```python
from build123d import *

# Parameters (mm, degrees)
EXTRUDE_1_DEPTH     = 5
FILLET_1_R          = 2.5
FILLET_2_R          = 1
EXTRUDE_2_DEPTH     = 8
FILLET_3_R          = 2.5
SKETCH_5_W          = 1.467751534
SKETCH_5_H          = 4.178210798
SKETCH_5_W_2        = 1.389566385
CUT_EXTRUDE_1_DEPTH = 20
FILLET_4_R          = 1.5
FILLET_5_R          = 1.5


with BuildPart() as part:
    # 草图1 → 凸台-拉伸1 (new body)
    with BuildSketch(Plane.XY):
        Polygon((0, 0), (0, 28), (4, 28), (7.380946094, 20.749537704), (11.912485029, 22.862629012), (7.185351304, 33), (-5, 33), (-5, -12), (-75, -12), (-75, -2), (-80, -2), (-80, -17), (0, -17), (0, -5), (8, -5), (8, 0), align=None)
    extrude(amount=EXTRUDE_1_DEPTH)

    # 圆角1
    fillet_1_edges = [part.edges().sort_by_distance(p)[0] for p in [
        (-77.5, -2, 0),
        (9.646715562, 21.806083358, 0),
        (9.646715562, 21.806083358, 5),
        (-80, -2, 2.5),
        (-75, -2, 2.5),
        (7.185351304, 33, 2.5),
        (11.912485029, 22.862629012, 2.5),
        (7.380946094, 20.749537704, 2.5),
        (-77.5, -2, 5),
    ]]
    fillet(fillet_1_edges, radius=FILLET_1_R - 0.0001)  # a hair under: the kernel refuses the full size

    # 圆角2
    fillet_2_edges = [part.edges().sort_by_distance(p)[0] for p in [
        (-5, 33, 2.5),
    ]]
    fillet(fillet_2_edges, radius=FILLET_2_R)

    # 草图3 → 凸台-拉伸2 (add)
    with BuildSketch(Plane(origin=(0, 0, 0), x_dir=(0, 0, -1), z_dir=(1, 0, 0))):
        with BuildLine():
            Line((-5, 0), (0, 0))
            ThreePointArc((0, 0), (-2.5, 2.5), (-5, 0))
        make_face()
    extrude(amount=EXTRUDE_2_DEPTH)

    # 圆角3
    fillet_3_edges = [part.edges().sort_by_distance(p)[0] for p in [
        (8, -2.5, 0),
        (8, -5, 2.5),
        (8, -2.5, 5),
        (8, 2.5, 2.5),
    ]]
    fillet(fillet_3_edges, radius=FILLET_3_R - 0.0001)  # a hair under: the kernel refuses the full size

    # 草图4 → 旋转3 (revolve)
    with BuildSketch(Plane(origin=(4.4, 0, 0), x_dir=(0, 0, -1), z_dir=(1, 0, 0))):
        with BuildLine():
            Line((-5.5, 0), (0.5, 0))
            ThreePointArc((0.5, 0), (-2.5, 3), (-5.5, 0))
        make_face()
    revolve(axis=Axis((4.4, 0, 2.5), (0, 0, -1)))

    # 草图5 → 切除-拉伸1 (cut)
    with BuildSketch(Plane.ZY.offset(5)):
        with Locations((-0.733875767, -0.010051234)):
            Rectangle(SKETCH_5_W, SKETCH_5_H)
        with Locations((5.694783193, -0.010051234)):
            Rectangle(SKETCH_5_W_2, SKETCH_5_H)
    extrude(amount=-CUT_EXTRUDE_1_DEPTH, mode=Mode.SUBTRACT)

    # 圆角4
    fillet_4_edges = [part.edges().sort_by_distance(p)[0] for p in [
        (-75, -12, 2.5),
        (-5, -12, 2.5),
    ]]
    fillet(fillet_4_edges, radius=FILLET_4_R)

    # 圆角5
    fillet_5_edges = [part.edges().sort_by_distance(p)[0] for p in [
        (0, -17, 2.5),
        (-80, -17, 2.5),
    ]]
    fillet(fillet_5_edges, radius=FILLET_5_R)


solid = part.part
```
The model under review builds one solid part; all positions refer to its coordinate system, in mm. A direction names the side the tool comes from. Give positions to 0.01 mm unless a question says otherwise; leave off trailing zeros. Write each loop counter-clockwise with the first axis right and the second up, starting at its lowest first coordinate (ties: lowest second). Pieces come first, ordered by that corner, then holes.
(1) To check wall thickness, follow L1, parallel to X at y = -9.5, z = 4.75; L2, parallel to Y at x = -63, z = 4.2; L3, parallel to X at y = 9, z = 2.9. State the ranges of each line that lie inside material, in increasing order.
(2) Consider section A-A, the plane x = -18. Give the boundary of the cut face in (y, z).
(3) Tool access review of faces 4 (the flat face through (-75, -8, 2)), 5 (the flat face through (2, 28, 2)), 6 (the cylindrical face through (-77.5, -3, 4.5)), 7 (the cylindrical face through (-77.5, -3, 0.5)), 8 (the cylindrical face through (7.248, -1.979, 4.287)): name each direction out of +Z, -Z, +X, -X, +Y, -Y from which nothing blocks a thin tool from reaching the whole face with its end or side.
(4) The part is to be moulded in two halves that separate along X. For faces 1 (the cylindrical face through (-79.5, -3, 2.5)), 2 (the flat face through (3, -5, 2)), 3 (the cylindrical face through (-75.436, -3.089, 2.535)), say which applies: released by +X, released by -X, zero draft, split by the parting line, or undercut.
(5) For P1, Ø2, axis at y = 10.5, z = 1.5, coming from the +X side; P2, Ø2.5, axis at x = 3.5, z = 2, coming from the -Y side; P3, Ø3, axis at y = 3.5, z = 3, coming from the -X side, all flat-tipped, find the tip position at first contact; note any pin that passes through.
(6) Consider section B-B, the plane y = 14.5. Give the boundary of the cut face in (x, z), and give its area (3 significant figures).
Returned:
1. L1: x = -80 to -75, -5 to 0
1. L2: y = -17 to -12
1. L3: x = -5 to 0
2. outline: (-17, 0) - (-12, 0) - (-12, 5) - (-17, 5) - close
3. face 4: +Z, -Z, +Y
3. face 5: +Z, -Z
3. face 6: +Z, -X, +Y
3. face 7: -Z, -X, +Y
3. face 8: +Z, +X, -Y
4. face 1: released by -X
4. face 2: zero draft
4. face 3: undercut
5. P1: stops at x = 0
5. P2: stops at y = -5
5. P3: stops at x = -5
6. outline: (-5, 0) - (0, 0) - (0, 5) - (-5, 5) - close
6. area: 25.0 mm2
